Could you check a few things on this drawing? It's one solid part, dimensions in mm from its lowest x, y, z. A direction names the side the tool comes from. Give positions to 0.01 mm unless a question says otherwise; leave off trailing zeros. Order: outer loops, then holes, each group sorted by start corner. A loop starts at its lowest first (then second) coordinate and runs counter-clockwise, first axis right, second up. Notation, with made-up numbers: M 14,32 L 58,32 A6 ccw 58,40 Z; hole C -16,80 d9. An arc over 180 degrees is marked long. Use one line per item in the form item = value. Start each with the question number.
1. Will these pins go through, and if not, where does the flat tip stop? P1, Ø3, axis at y = 15.5, z = 23.5, coming from the +X side; P2, Ø1, axis at x = 3.5, z = 11, coming from the -Y side; P3, Ø1.5, axis at x = 3, z = 2, coming from the +Y side; P4, Ø0.9, axis at y = 8.5, z = 26.5, coming from the -X side.
2. I want a section at A-A, the plane x = 3.55. List the corners of the cut face in (y, z) for me, and give its area (3 significant figures).
3. We'd pull the mould along Z, two halves only. Please class the marked faces 3, 4, 5 and 6: +Z half, -Z half, draft (parallel to the pull), parting line (faces both ways), or undercut.
4. For the marked faces 1 and 2, which set-ups out of +Z, -Z, +X, -X, +Y, -Y let a thin tool reach every point of the face, with its end or its side?
5. I want a section at D-D, the plane y = 14.5. List the corners of the cut face in (x, z) for me.
6. I want a section at C-C, the plane z = 9.5. List the corners of the cut face in (x, y) for me.
7. I want a section at B-B, the plane y = 2.5. List the corners of the cut face in (x, z) for me.
8. I need wall thicknesses on L1, parallel to Z at x = 0.65, y = 15.5; L2, parallel to Y at x = 1.55, z = 1.75; L3, parallel to X at y = 5.25, z = 1. Which ranges of each line are inside material? Lowest first, please.
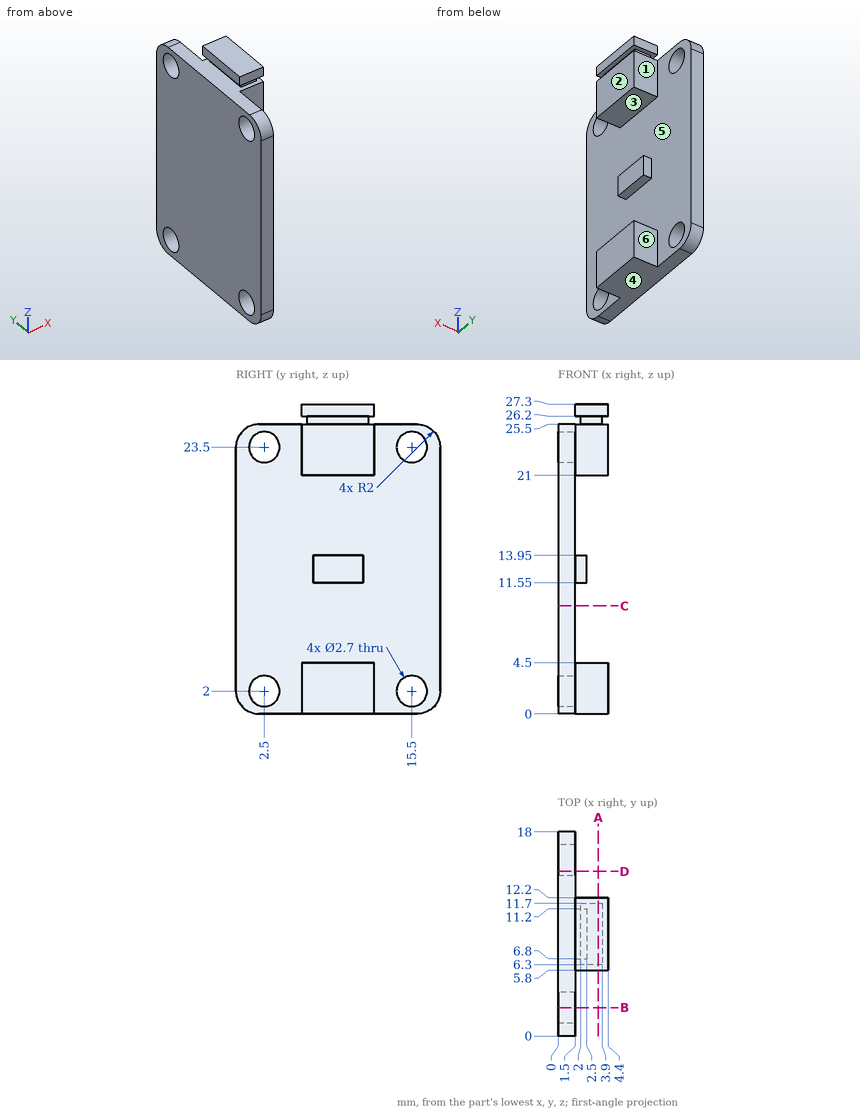
Check result:
q1.P1 = 1.5
q1.P2 = through
q1.P3 = 12.2
q1.P4 = 1.5
q2.outline = M 5.8,0 L 12.2,0 L 12.2,4.5 L 5.8,4.5 Z; M 5.8,21 L 12.2,21 L 12.2,25.5 L 11.7,25.5 L 11.7,26.2 L 12.2,26.2 L 12.2,27.3 L 5.8,27.3 L 5.8,26.2 L 6.3,26.2 L 6.3,25.5 L 5.8,25.5 Z
q2.area = 68.4 mm2
q3.face_3 = undercut
q3.face_4 = -Z half
q3.face_5 = undercut
q3.face_6 = draft
q4.face_1 = +Z, -Z, +X, +Y
q4.face_2 = +Z, -Z, +X, +Y, -Y
q5.outline = M 0,0 L 1.5,0 L 1.5,1.09 L 0,1.09 Z; M 0,2.91 L 1.5,2.91 L 1.5,22.59 L 0,22.59 Z; M 0,24.41 L 1.5,24.41 L 1.5,25.5 L 0,25.5 Z
q6.outline = M 0,0 L 1.5,0 L 1.5,18 L 0,18 Z
q7.outline = M 0,0 L 1.5,0 L 1.5,0.65 L 0,0.65 Z; M 0,3.35 L 1.5,3.35 L 1.5,22.15 L 0,22.15 Z; M 0,24.85 L 1.5,24.85 L 1.5,25.5 L 0,25.5 Z
q8.L1 = 0 to 0.65, 3.35 to 22.15, 24.85 to 25.5
q8.L2 = 5.8 to 12.2
q8.L3 = 0 to 1.5
